from build123d import *

# Parameters (mm, degrees)
F1_DEPTH = 34
F0_R     = 61
F0_R_2   = 59
F0_R_3   = 56.5
F0_R_4   = 54.5
F2_DEPTH = 3
F3_START = 34
F0_R_5   = 14.5
F3_DEPTH = 3
F4_DEPTH = 6
F6_DEPTH = 61.001


with BuildPart() as f1:
    # F0 (on Top) → F1 (new body)
    with BuildSketch(Plane.XY):
        with BuildLine():
            ThreePointArc((-17.5, 0), (0, 17.5), (17.5, 0))
            ThreePointArc((17.5, 0), (18.25, 0.75), (19, 0))
            ThreePointArc((19, 0), (-2.7e-09, 19), (-19, -5.4e-09))
            ThreePointArc((-19, -5.4e-09), (-18.2500000027, 0.75), (-17.5, 0))
        make_face()
        with BuildLine():
            ThreePointArc((19, 0), (18.25, 0.75), (17.5, 0))
            ThreePointArc((17.5, 0), (18.25, -0.75), (19, 0))
        make_face()
        with BuildLine():
            ThreePointArc((-19, -5.4e-09), (-18.2499999973, -0.75), (-17.5, 0))
            ThreePointArc((-17.5, 0), (-18.2500000027, 0.75), (-19, -5.4e-09))
        make_face()
    extrude(amount=F1_DEPTH)

    # F0 (on Top) → F2 (join)
    with BuildSketch(Plane.XY):
        Circle(F0_R)
        Circle(F0_R_2, mode=Mode.SUBTRACT)
        Circle(F0_R_2)
        Circle(F0_R_3, mode=Mode.SUBTRACT)
        Circle(F0_R_3)
        Circle(F0_R_4, mode=Mode.SUBTRACT)
        Circle(F0_R_4)
        with BuildLine():
            ThreePointArc((-19, -5.4e-09), (-2.7e-09, 19), (19, 0))
            ThreePointArc((19, 0), (2.7e-09, -19), (-19, -5.4e-09))
        make_face(mode=Mode.SUBTRACT)
    extrude(amount=F2_DEPTH)

    # F0 (on Top) → F3 (join)
    with BuildSketch(Plane.XY.offset(F3_START)):
        with BuildLine():
            ThreePointArc((-17.5, 0), (0, -17.5), (17.5, 0))
            ThreePointArc((17.5, 0), (0, 17.5), (-17.5, 0))
        make_face()
        Circle(F0_R_5, mode=Mode.SUBTRACT)
        with BuildLine():
            ThreePointArc((-17.5, 0), (0, 17.5), (17.5, 0))
            ThreePointArc((17.5, 0), (18.25, 0.75), (19, 0))
            ThreePointArc((19, 0), (-2.7e-09, 19), (-19, -5.4e-09))
            ThreePointArc((-19, -5.4e-09), (-18.2500000027, 0.75), (-17.5, 0))
        make_face()
        with BuildLine():
            ThreePointArc((19, 0), (18.25, 0.75), (17.5, 0))
            ThreePointArc((17.5, 0), (18.25, -0.75), (19, 0))
        make_face()
        with BuildLine():
            ThreePointArc((-19, -5.4e-09), (-18.2499999973, -0.75), (-17.5, 0))
            ThreePointArc((-17.5, 0), (-18.2500000027, 0.75), (-19, -5.4e-09))
        make_face()
        with BuildLine():
            ThreePointArc((19, 0), (18.25, -0.75), (17.5, 0))
            ThreePointArc((17.5, 0), (0, -17.5), (-17.5, 0))
            ThreePointArc((-17.5, 0), (-18.2499999973, -0.75), (-19, -5.4e-09))
            ThreePointArc((-19, -5.4e-09), (2.7e-09, -19), (19, 0))
        make_face()
    extrude(amount=F3_DEPTH)

    # F0 (on Top) → F4 (join)
    with BuildSketch(Plane.XY):
        Circle(F0_R)
        Circle(F0_R_2, mode=Mode.SUBTRACT)
        Circle(F0_R_3)
        Circle(F0_R_4, mode=Mode.SUBTRACT)
    extrude(amount=F4_DEPTH)

    # F5 (on Front) → F6 (cut, through all)
    with BuildSketch(Plane.XZ):
        Polygon((-20, 6), (0, 3), (0, 6), align=None)
        Polygon((0, 6), (0, 3), (20, 6), align=None)
    extrude(amount=F6_DEPTH, mode=Mode.SUBTRACT)


solid = f1.part
Here's how the part is built. I have some questions about the finished solid (model axes, mm). A direction names the side the tool comes from. Coordinates: 2 decimals unless noted, no trailing zeros. Write each loop counter-clockwise with the first axis right and the second up, starting at its lowest first coordinate (ties: lowest second). Pieces come first, ordered by that corner, then holes.
Item 1: I want a section at C-C on z = 20. Write out the boundary of the cut face in (x, y), and give its area (3 significant figures).
Item 2: If we mould it in two halves opening along X, with no side actions, what happens to faces 5 (the flat face through (-1, -23, 3)), 6 (the flat face through (-10, -58.9, 4.5)), 7 (the flat face through (13, 14, 0)), 8 (the cylindrical face through (-7.94, 60.48, 2.96))? For each: +X half, -X half, draft (parallel to the pull), parting line (faces both ways), or undercut.
Item 3: I want a section at A-A on y = 16. Write out the boundary of the cut face in (x, z).
Item 4: I want a section at D-D on y = -12. Write out the boundary of the cut face in (x, z), and give its area (3 significant figures).
Item 5: If I drill on line 1 (Y direction, x = 0, z = 36); line 2 (Y direction, x = 1, z = 33); line 3 (Z direction, x = 23.5, y = 51.5), over which ranges is the centre line in solid material (lowest first)?
Item 6: Will these pins go through, and if not, where does the flat tip stop? pin 1 (6 mm diameter, centred on x = -27.5, y = 14.5, fed in from +Z); pin 2 (6 mm diameter, centred on x = 30.5, y = 47, fed in from -Z); pin 3 (8 mm diameter, centred on x = -14, y = -4, fed in from -Z); pin 4 (1 mm diameter, centred on y = 16.5, z = 16, fed in from -X).
Item 7: I want a section at B-B on x = 48. Write out the boundary of the cut face in (y, z).
Item 8: On a 3-axis mill with a long thin cutter (end or side, diameter ignored), from which of +Z, -Z, +X, -X, +Y, -Y can I reach the whole of each face in a straight line? I mean faces 1 (the flat face through (0, -57, 3)), 2 (the flat face through (-4.3, -14.2, 34)), 3 (the cylindrical face through (-0.385, 17.496, 16.762)), 4 (the flat face through (-10, -54, 4.5)). Say none if no direction works.
Findings below:
1. outline: (-19, 0) arc R0.75 ccw to (-17.5, 0) arc R17.5 cw to (17.5, 0) arc R0.75 ccw to (19, 0) arc R19 ccw to start
1. area: 87.8 mm2
2. face 5: undercut
2. face 6: undercut
2. face 7: draft
2. face 8: parting line
3. outline: (-58.86, 0) - (-7.09, 0) - (-7.09, 34) - (7.09, 34) - (7.09, 0) - (58.86, 0) - (58.86, 6) - (56.79, 6) - (56.79, 3) - (54.19, 3) - (54.19, 6) - (52.1, 6) - (52.1, 3) - (10.25, 3) - (10.25, 37) - (-10.25, 37) - (-10.25, 3) - (-52.1, 3) - (-52.1, 6) - (-54.19, 6) - (-54.19, 3) - (-56.79, 3) - (-56.79, 6) - (-58.86, 6) - close
4. outline: (-59.81, 0) - (-14.73, 0) - (-14.73, 3) - (-53.16, 3) - (-53.16, 6) - (-55.21, 6) - (-55.21, 3) - (-57.77, 3) - (-57.77, 6) - (-59.81, 6) - close; (-14.73, 34) - (-8.14, 34) - (-8.14, 37) - (-14.73, 37) - close; (8.14, 34) - (14.73, 34) - (14.73, 37) - (8.14, 37) - close; (14.73, 0) - (59.81, 0) - (59.81, 6) - (57.77, 6) - (57.77, 3) - (55.21, 3) - (55.21, 6) - (53.16, 6) - (53.16, 3) - (14.73, 3) - close
4. area: 335 mm2
5. line 1: y = -19 to -14.5, 14.5 to 19
5. line 2: y = 17.47 to 18.97
5. line 3: z = 0 to 3
6. pin 1: stops at z = 3
6. pin 2: stops at z = 0
6. pin 3: stops at z = 34
6. pin 4: stops at x = -10.25
7. outline: (-37.64, 0) - (37.64, 0) - (37.64, 6) - (34.31, 6) - (34.31, 3) - (29.8, 3) - (29.8, 6) - (25.81, 6) - (25.81, 3) - (-25.81, 3) - (-25.81, 6) - (-29.8, 6) - (-29.8, 3) - (-34.31, 3) - (-34.31, 6) - (-37.64, 6) - close
8. face 1: +Z
8. face 2: -Z, -Y
8. face 3: -Z
8. face 4: +Z, -Y
